from build123d import *

# Parameters (mm, degrees)
SKETCH1_W           = 305
SKETCH1_H           = 290
SKETCH1_R           = 17.5
SKETCH1_R_2         = 2.5
SKETCH1_R_3         = 2
BOSS_EXTRUDE1_DEPTH = 10


with BuildPart() as part:
    # Sketch1 → Boss-Extrude1 (new body)
    with BuildSketch(Plane(origin=(0, 0, 0), x_dir=(1, 0, 0), z_dir=(0, 1, 0))):
        with Locations((-22.5, 0)):
            Rectangle(SKETCH1_W, SKETCH1_H)
        with Locations((25, 0)):
            Circle(SKETCH1_R, mode=Mode.SUBTRACT)
        with Locations((95, 0)):
            Circle(SKETCH1_R_2, mode=Mode.SUBTRACT)
        with Locations((56.819805153, 31.819805153)):
            Circle(SKETCH1_R_3, mode=Mode.SUBTRACT)
        with Locations((60, -60.621778265)):
            Circle(SKETCH1_R_2, mode=Mode.SUBTRACT)
        with Locations((-10, -60.621778265)):
            Circle(SKETCH1_R_2, mode=Mode.SUBTRACT)
        with Locations((-45, 0)):
            Circle(SKETCH1_R_2, mode=Mode.SUBTRACT)
        with Locations((56.819805153, -31.819805153)):
            Circle(SKETCH1_R_3, mode=Mode.SUBTRACT)
        with Locations((-6.819805153, -31.819805153)):
            Circle(SKETCH1_R_3, mode=Mode.SUBTRACT)
        with Locations((-6.819805153, 31.819805153)):
            Circle(SKETCH1_R_3, mode=Mode.SUBTRACT)
        with Locations((-165, 0)):
            Circle(SKETCH1_R_2, mode=Mode.SUBTRACT)
        with Locations((-75, -135)):
            Circle(SKETCH1_R_2, mode=Mode.SUBTRACT)
        with Locations((95, -135)):
            Circle(SKETCH1_R_2, mode=Mode.SUBTRACT)
        with Locations((95, 135)):
            Circle(SKETCH1_R_2, mode=Mode.SUBTRACT)
        with Locations((-75, 135)):
            Circle(SKETCH1_R_2, mode=Mode.SUBTRACT)
        with Locations((-10, 60.621778265)):
            Circle(SKETCH1_R_2, mode=Mode.SUBTRACT)
        with Locations((60, 60.621778265)):
            Circle(SKETCH1_R_2, mode=Mode.SUBTRACT)
    extrude(amount=BOSS_EXTRUDE1_DEPTH)


solid = part.part
Build history of the part. All positions in model axes, mm. Round coordinates to 2 decimals unless told otherwise and drop trailing zeros. Loops run counter-clockwise (first coordinate to the right, second up) from the corner with the lowest first, then second, coordinate; pieces in that order, holes last. Notation, with made-up numbers: (20.5, -8) -> (49.5, -8) arc R19 ccw to (49.5, 24) -> close; hole circle Ø9 at (61.25, -8.5). An arc over 180 degrees is marked (long way). One line per item, written item: value. Start each with the question number.
Q1. Probe line 1 along X through (y, z) = (6.25, 32); line 2 along X through (y, z) = (6, 0); line 3 along Z through (x, y) = (-45, 7). List the from-to ranges inside material, lowest first.
Q2. Two-plate mould, pull along Z, no slides. Class faces 1 (the face through (-25, 5, -145)), 2 (the face through (-175, 5, 2)), 3 (the face through (11.113, 4.93, 10.648)): released by +Z, released by -Z, zero draft, split by the parting line, or undercut.
Q3. Cut at A-A on x = 25. List the corners of the cut face in (y, z), plus the area to 3 significant figures.
Computed:
1. line 1: -175 to -8.81, -4.83 to 54.83, 58.81 to 130
1. line 2: -175 to -167.5, -162.5 to -47.5, -42.5 to 7.5, 42.5 to 92.5, 97.5 to 130
1. line 3: -145 to -2.5, 2.5 to 145
2. face 1: released by -Z
2. face 2: zero draft
2. face 3: undercut
3. outline: (0, -145) -> (10, -145) -> (10, -17.5) -> (0, -17.5) -> close; (0, 17.5) -> (10, 17.5) -> (10, 145) -> (0, 145) -> close
3. area: 2,550 mm²
